Part model, mm, in its own coordinate system. A direction names the side the tool comes from. Give positions to 0.01 mm unless a question says otherwise; leave off trailing zeros. Write each loop counter-clockwise with the first axis right and the second up, starting at its lowest first coordinate (ties: lowest second). Pieces come first, ordered by that corner, then holes. Notation, with made-up numbers: M 50.25,38.5 L 96.25,38.5 A26 cw 96.25,77.5 Z; hole C 59,-29 d6. An arc over 180 degrees is marked long. Answer as CSV lines item,"result". Start each with the question number.
1) Wall check: line 1 along Z through (x, y) = (-0.25, -4); line 2 along X through (y, z) = (2.4, 20); line 3 along Z through (x, y) = (-2, -1.5). Give the ranges that are in metal, low to high. Write a range as from..to.
2) Slice it at A-A, the plane x = 0. Give the cut face in (y, z), plus the area to 3 significant figures.
3) Mould opens along X. For faces 1 (the flat face through (-2, 0.221, 22)), 2 (the flat face through (-10.356, 3, 49)), 3 (the flat face through (0, 0, 0)) say: pulls with the +X half, pulls with the -X half, needs draft (parallel to the pull), parting line crosses it, or undercut.
4) Tool access for faces 4 (the cylindrical face through (-1.436, 2.788, 83.464)), 5 (the flat face through (-9.486, 1.315, 49.3)), 6 (the flat face through (9.46, 1.29, 49.3)): list every direction of +Z, -Z, +X, -X, +Y, -Y with a clear straight run to the whole face (end or side of a thin tool).
5) Pin check, flat tips, straight feed: pin 1 Ø2 at (x, z) = (-1, 81.5) entering from +Y; pin 2 Ø0.7 at (y, z) = (0, 74) entering from +X; pin 3 Ø0.5 at (x, z) = (9.5, 34.5) entering from +Y. Stop position of each tip, or through.
6) Slice it at C-C, the plane z = 65. Give the cut face in (x, y), plus the area to 3 significant figures.
```python
from build123d import *

# Parameters (mm, degrees)
BOSS_EXTRUDE1_DEPTH = 100
SKETCH2_R           = 3.75
CUT_EXTRUDE1_DEPTH  = 5.064116728
SKETCH3_R           = 2.25
CUT_EXTRUDE2_DEPTH  = 101.674424562


with BuildPart() as part:
    # Sketch1 → Boss-Extrude1 (new body)
    with BuildSketch(Plane.XY):
        Polygon((-10.313155992, -4.579057074), (-10.313155992, -5.079057074), (10.313155992, -5.079057074), (10.313155992, -4.579057074), (9.554252946, -3.820154028), (10.356146045, -3.018260929), (10.356146045, -2.320637728), (9.927498969, -1.891990652), (9.459466628, -1.891990652), (8.591867013, -1.024391036), (8.591867013, 0.420032401), (10.356146045, 2.184311433), (10.356146045, 3.776726056), (8.847812446, 5.285059654), (-8.847812446, 5.285059654), (-10.356146045, 3.776726056), (-10.356146045, 2.184311433), (-8.591867013, 0.420032401), (-8.591867013, -1.024391036), (-9.459466628, -1.891990652), (-9.927498969, -1.891990652), (-10.356146045, -2.320637728), (-10.356146045, -3.018260929), (-9.554252946, -3.820154028), align=None)
    extrude(amount=BOSS_EXTRUDE1_DEPTH)

    # Sketch2 → Cut-Extrude1 (cut)
    with BuildSketch(Plane(origin=(0, 5.285059654, 0), x_dir=(1, 0, 0), z_dir=(0, 1, 0))):
        with Locations(Location((0, -20, 0), (0, 0, 270))):
            Circle(SKETCH2_R)
        with Locations(Location((0, -80, 0), (0, 0, 270))):
            Circle(SKETCH2_R)
    extrude(amount=-CUT_EXTRUDE1_DEPTH, mode=Mode.SUBTRACT)

    # Sketch3 → Cut-Extrude2 (cut, through all)
    with BuildSketch(Plane(origin=(0, 0.220942926, 0), x_dir=(1, 0, 0), z_dir=(0, 1, 0))):
        with Locations(Location((0, -20, 0), (0, 0, 270))):
            Circle(SKETCH3_R)
        with Locations(Location((0, -80, 0), (0, 0, 270))):
            Circle(SKETCH3_R)
    extrude(amount=-CUT_EXTRUDE2_DEPTH, mode=Mode.SUBTRACT)


solid = part.part
```
Found:
1,line 1,"0..17.76, 22.24..77.76, 82.24..100"
1,line 2,"-10.36..-3.75, 3.75..10.36"
1,line 3,"0..18.97, 21.03..78.97, 81.03..100"
2,outline,"M -5.08,0 L 5.29,0 L 5.29,16.25 L 0.22,16.25 L 0.22,17.75 L -5.08,17.75 Z; M -5.08,22.25 L 0.22,22.25 L 0.22,23.75 L 5.29,23.75 L 5.29,76.25 L 0.22,76.25 L 0.22,77.75 L -5.08,77.75 Z; M -5.08,82.25 L 0.22,82.25 L 0.22,83.75 L 5.29,83.75 L 5.29,100 L -5.08,100 Z"
2,area,"913 mm²"
3,face 1,"undercut"
3,face 2,"pulls with the -X half"
3,face 3,"needs draft"
4,face 4,"+Y"
4,face 5,"+Z, -Z, -X"
4,face 6,"+Z, -Z, +X"
5,pin 1,"y = 0.22"
5,pin 2,"x = 8.59"
5,pin 3,"y = 4.88"
6,outline,"M -10.36,-3.02 L -9.55,-3.82 L -10.31,-4.58 L -10.31,-5.08 L 10.31,-5.08 L 10.31,-4.58 L 9.55,-3.82 L 10.36,-3.02 L 10.36,-2.32 L 9.93,-1.89 L 9.46,-1.89 L 8.59,-1.02 L 8.59,0.42 L 10.36,2.18 L 10.36,3.78 L 8.85,5.29 L -8.85,5.29 L -10.36,3.78 L -10.36,2.18 L -8.59,0.42 L -8.59,-1.02 L -9.46,-1.89 L -9.93,-1.89 L -10.36,-2.32 Z"
6,area,"200 mm²"
